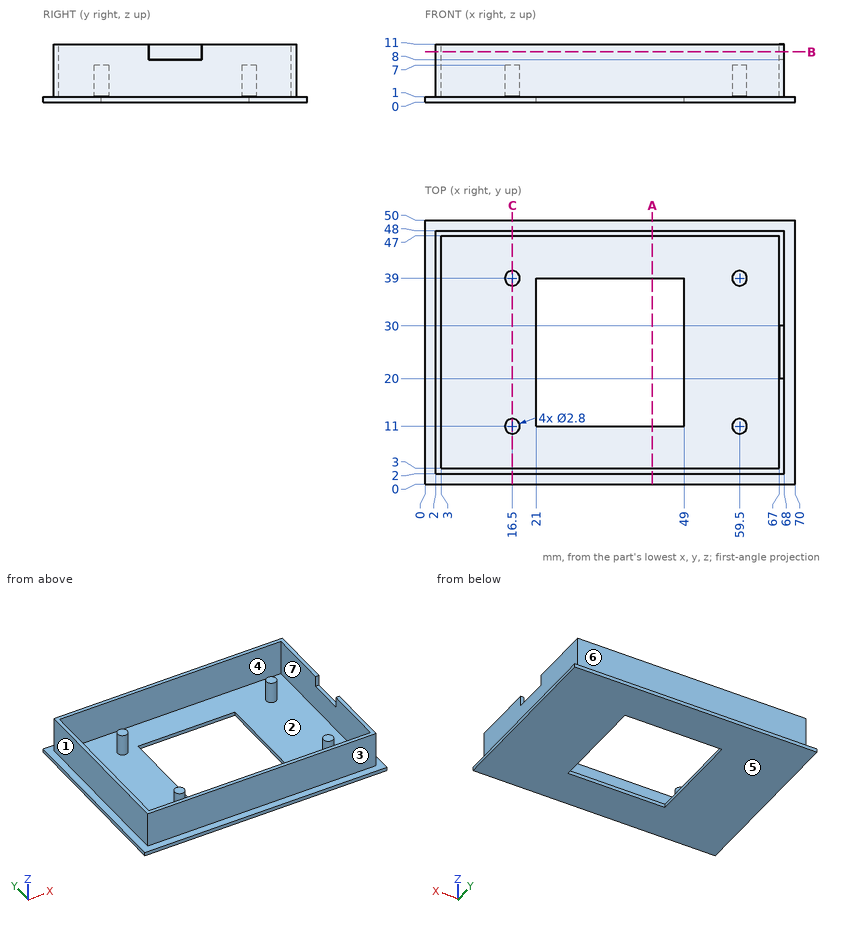
Here's the drawing with two shaded views (mm, measured from the low corner). I have some questions. A direction names the side the tool comes from. Give positions to 0.01 mm unless a question says otherwise; leave off trailing zeros. Loops run counter-clockwise (first coordinate to the right, second up) from the corner with the lowest first, then second, coordinate; pieces in that order, holes last. Notation, with made-up numbers: (38, -14.5) - (43, -14.5) arc R13 ccw to (43, -6.5) - close; hole circle Ø5 at (31.5, -14). An arc over 180 degrees is marked (long way). One line per item, written item: value.
(1) I need wall thicknesses on line 1 along Y through (x, z) = (15, 9.25); line 2 along X through (y, z) = (11, 8.5); line 3 along Z through (x, y) = (57, 16.5). Which ranges of each line are inside material? Lowest first, please.
Verdict:
line 1: 2 to 3, 47 to 48
line 2: 2 to 3, 67 to 68
line 3: 0 to 1
(2) On a 3-axis mill with a long thin cutter (end or side, diameter ignored), from which of +Z, -Z, +X, -X, +Y, -Y can I reach the whole of each face in a straight line? I mean the marked faces 5, 6 and 7. Say none if no direction works.
Verdict:
face 5: -Z, +X, -X, +Y, -Y
face 6: +Z, +X, -X, +Y
face 7: +Z
(3) I'm going to push flat-ended pins straight in: pin 1 (3 mm diameter, centred on x = 32.5, y = 44, fed in from +Z); pin 2 (1 mm diameter, centred on x = 55, y = 9, fed in from -Z); pin 3 (0.8 mm diameter, centred on x = 67.5, z = 10, fed in from +Y); pin 4 (2 mm diameter, centred on x = 60, y = 39, fed in from +Z). Where does each tip first touch, or does it pass through?
Verdict:
pin 1: z = 1
pin 2: z = 0
pin 3: y = 48
pin 4: z = 7
(4) If we section it at B-B, the plane z = 9.5: List the corners of the cut face in (x, y) for me.
Verdict:
outline: (2, 2) - (68, 2) - (68, 20) - (67, 20) - (67, 3) - (3, 3) - (3, 47) - (67, 47) - (67, 30) - (68, 30) - (68, 48) - (2, 48) - close
(5) If we section it at A-A, the plane x = 43: List the corners of the cut face in (y, z) for me, plus the area to 3 significant figures.
Verdict:
outline: (0, 0) - (11, 0) - (11, 1) - (3, 1) - (3, 11) - (2, 11) - (2, 1) - (0, 1) - close; (39, 0) - (50, 0) - (50, 1) - (48, 1) - (48, 11) - (47, 11) - (47, 1) - (39, 1) - close
area: 42.0 mm^2
(6) If we mould it in two halves opening along Y, with no side actions, what happens to the marked faces 1, 2, 3 and 4? For each: released by +Y, released by -Y, zero draft, split by the parting line, or undercut.
Verdict:
face 1: zero draft
face 2: undercut
face 3: released by -Y
face 4: undercut
(7) If we section it at C-C, the plane x = 16.5: List the corners of the cut face in (y, z) for me.
Verdict:
outline: (0, 0) - (50, 0) - (50, 1) - (48, 1) - (48, 11) - (47, 11) - (47, 1) - (40.4, 1) - (40.4, 7) - (37.6, 7) - (37.6, 1) - (12.4, 1) - (12.4, 7) - (9.6, 7) - (9.6, 1) - (3, 1) - (3, 11) - (2, 11) - (2, 1) - (0, 1) - close
